```python
from build123d import *

# Parameters (mm, degrees)
F0_W     = 63.8
F0_H     = 39.8
F0_W_2   = 41
F0_H_2   = 20.8
F1_DEPTH = 3.8
F3_DEPTH = 25


with BuildPart() as f1:
    # F0 (on Front) → F1 (new body)
    with BuildSketch(Plane.XZ):
        Rectangle(F0_W, F0_H)
        Rectangle(F0_W_2, F0_H_2, mode=Mode.SUBTRACT)
    extrude(amount=F1_DEPTH)

    # F2 (on face) → F3 (cut)
    with BuildSketch(Plane.XZ.offset(3.8)):
        Polygon((-29.2, 17.2), (-30.8, 17.2), (-30.8, 14.8), (-29.2, 14.8), (-29.2, 13.2), (-26.8, 13.2), (-26.8, 14.8), (-25.2, 14.8), (-25.2, 17.2), (-26.8, 17.2), (-26.8, 18.8), (-29.2, 18.8), align=None)
        Polygon((-26.8, -13.2), (-29.2, -13.2), (-29.2, -14.8), (-30.8, -14.8), (-30.8, -17.2), (-29.2, -17.2), (-29.2, -18.8), (-26.8, -18.8), (-26.8, -17.2), (-25.2, -17.2), (-25.2, -14.8), (-26.8, -14.8), align=None)
        Polygon((-18.8, 18.8), (-21.2, 18.8), (-21.2, 17.2), (-22.8, 17.2), (-22.8, 14.8), (-21.2, 14.8), (-21.2, 13.2), (-18.8, 13.2), (-18.8, 14.8), (-17.2, 14.8), (-17.2, 17.2), (-18.8, 17.2), align=None)
        Polygon((-18.8, -13.2), (-21.2, -13.2), (-21.2, -14.8), (-22.8, -14.8), (-22.8, -17.2), (-21.2, -17.2), (-21.2, -18.8), (-18.8, -18.8), (-18.8, -17.2), (-17.2, -17.2), (-17.2, -14.8), (-18.8, -14.8), align=None)
        Polygon((-10.8, 18.8), (-13.2, 18.8), (-13.2, 17.2), (-14.8, 17.2), (-14.8, 14.8), (-13.2, 14.8), (-13.2, 13.2), (-10.8, 13.2), (-10.8, 14.8), (-9.2, 14.8), (-9.2, 17.2), (-10.8, 17.2), align=None)
        Polygon((-10.8, -13.2), (-13.2, -13.2), (-13.2, -14.8), (-14.8, -14.8), (-14.8, -17.2), (-13.2, -17.2), (-13.2, -18.8), (-10.8, -18.8), (-10.8, -17.2), (-9.2, -17.2), (-9.2, -14.8), (-10.8, -14.8), align=None)
        Polygon((-2.8, 18.8), (-5.2, 18.8), (-5.2, 17.2), (-6.8, 17.2), (-6.8, 14.8), (-5.2, 14.8), (-5.2, 13.2), (-2.8, 13.2), (-2.8, 14.8), (-1.2, 14.8), (-1.2, 17.2), (-2.8, 17.2), align=None)
        Polygon((-2.8, -13.2), (-5.2, -13.2), (-5.2, -14.8), (-6.8, -14.8), (-6.8, -17.2), (-5.2, -17.2), (-5.2, -18.8), (-2.8, -18.8), (-2.8, -17.2), (-1.2, -17.2), (-1.2, -14.8), (-2.8, -14.8), align=None)
        Polygon((5.2, 18.8), (2.8, 18.8), (2.8, 17.2), (1.2, 17.2), (1.2, 14.8), (2.8, 14.8), (2.8, 13.2), (5.2, 13.2), (5.2, 14.8), (6.8, 14.8), (6.8, 17.2), (5.2, 17.2), align=None)
        Polygon((5.2, -13.2), (2.8, -13.2), (2.8, -14.8), (1.2, -14.8), (1.2, -17.2), (2.8, -17.2), (2.8, -18.8), (5.2, -18.8), (5.2, -17.2), (6.8, -17.2), (6.8, -14.8), (5.2, -14.8), align=None)
        Polygon((13.2, 18.8), (10.8, 18.8), (10.8, 17.2), (9.2, 17.2), (9.2, 14.8), (10.8, 14.8), (10.8, 13.2), (13.2, 13.2), (13.2, 14.8), (14.8, 14.8), (14.8, 17.2), (13.2, 17.2), align=None)
        Polygon((13.2, -13.2), (10.8, -13.2), (10.8, -14.8), (9.2, -14.8), (9.2, -17.2), (10.8, -17.2), (10.8, -18.8), (13.2, -18.8), (13.2, -17.2), (14.8, -17.2), (14.8, -14.8), (13.2, -14.8), align=None)
        Polygon((21.2, 18.8), (18.8, 18.8), (18.8, 17.2), (17.2, 17.2), (17.2, 14.8), (18.8, 14.8), (18.8, 13.2), (21.2, 13.2), (21.2, 14.8), (22.8, 14.8), (22.8, 17.2), (21.2, 17.2), align=None)
        Polygon((21.2, -13.2), (18.8, -13.2), (18.8, -14.8), (17.2, -14.8), (17.2, -17.2), (18.8, -17.2), (18.8, -18.8), (21.2, -18.8), (21.2, -17.2), (22.8, -17.2), (22.8, -14.8), (21.2, -14.8), align=None)
        Polygon((29.2, 18.8), (26.8, 18.8), (26.8, 17.2), (25.2, 17.2), (25.2, 14.8), (26.8, 14.8), (26.8, 13.2), (29.2, 13.2), (29.2, 14.8), (30.8, 14.8), (30.8, 17.2), (29.2, 17.2), align=None)
        Polygon((29.2, -13.2), (26.8, -13.2), (26.8, -14.8), (25.2, -14.8), (25.2, -17.2), (26.8, -17.2), (26.8, -18.8), (29.2, -18.8), (29.2, -17.2), (30.8, -17.2), (30.8, -14.8), (29.2, -14.8), align=None)
    extrude(amount=-F3_DEPTH, mode=Mode.SUBTRACT)


solid = f1.part
```
Source: CAD feature listing. Evaluate the final solid. Frame: model axes, mm. Round coordinates to 2 decimals unless told otherwise and drop trailing zeros. Loops run counter-clockwise (first coordinate to the right, second up) from the corner with the lowest first, then second, coordinate; pieces in that order, holes last.
1. Section query C-C on x = -3.5. Output: boundary loops of the cut face in (y, z), and give its area (3 significant figures).
2. Section query D-D on z = 15.5. Give the number of separate pieces and of enclosed holes in the cut face, and give its area (3 significant figures).
3. Mould query, pull axis Z, two halves, no side actions, for faces 1 (the flat face through (-6.8, -2, 16)), 2 (the flat face through (25.2, -2, 16)), 3 (the flat face through (0, -3.8, -13)). Classes: released by +Z, released by -Z, zero draft, split by the parting line, or undercut.
4. Section query B-B on z = 5. Output: boundary loops of the cut face in (x, y).
5. Section query A-A on x = -15.5. Output: boundary loops of the cut face in (y, z).
6. Ray query, L1, parallel to Z at x = 5, y = -0.65; L2, parallel to Z at x = 2, y = -3.1; L3, parallel to X at y = -1.95, z = 0.5. Return the intervals inside material, ascending.
Answers below:
1. outline: (-3.8, -19.9) - (0, -19.9) - (0, -18.8) - (-3.8, -18.8) - close; (-3.8, -13.2) - (0, -13.2) - (0, -10.4) - (-3.8, -10.4) - close; (-3.8, 10.4) - (0, 10.4) - (0, 13.2) - (-3.8, 13.2) - close; (-3.8, 18.8) - (0, 18.8) - (0, 19.9) - (-3.8, 19.9) - close
1. area: 29.6 mm2
2. separate pieces: 9
2. enclosed holes: 0
2. area: 72.2 mm2
3. face 1: undercut
3. face 2: undercut
3. face 3: zero draft
4. outline: (-31.9, -3.8) - (-20.5, -3.8) - (-20.5, 0) - (-31.9, 0) - close; (20.5, -3.8) - (31.9, -3.8) - (31.9, 0) - (20.5, 0) - close
5. outline: (-3.8, -19.9) - (0, -19.9) - (0, -10.4) - (-3.8, -10.4) - close; (-3.8, 10.4) - (0, 10.4) - (0, 19.9) - (-3.8, 19.9) - close
6. L1: z = -19.9 to -18.8, -13.2 to -10.4, 10.4 to 13.2, 18.8 to 19.9
6. L2: z = -19.9 to -17.2, -14.8 to -10.4, 10.4 to 14.8, 17.2 to 19.9
6. L3: x = -31.9 to -20.5, 20.5 to 31.9
